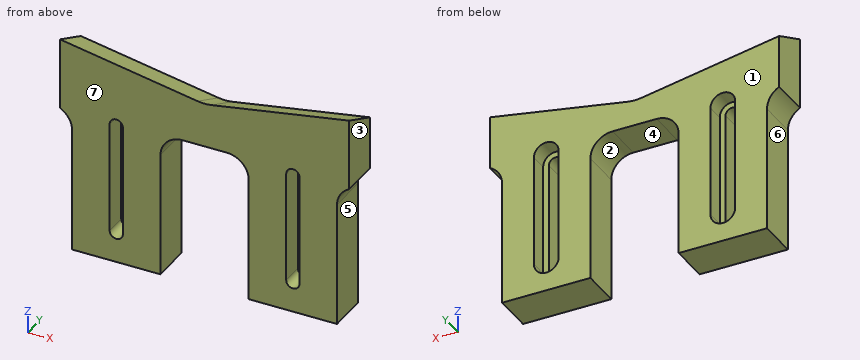
from build123d import *

# Parameters (mm, degrees)
BOSS_EXTRUDE1_DEPTH = 9
CUT_EXTRUDE2_REACH  = 93.001
SKETCH5_W           = 20
SKETCH5_H           = 33.343656478
SKETCH5_W_2         = 7.75
CUT_EXTRUDE3_DEPTH  = 10
FILLET1_R           = 5
CUT_EXTRUDE4_DEPTH  = 4
CHAMFER1_SIZE       = 9
CHAMFER1_SIZE_2     = 4.196768923
FILLET2_R           = 10
CUT_EXTRUDE5_REACH  = 93.001
SKETCH7_W           = 5
SKETCH7_H           = 18.120809616


with BuildPart() as part:
    # Sketch1 → Boss-Extrude1 (new body)
    with BuildSketch(Plane(origin=(0, 0, 0), x_dir=(1, 0, 0), z_dir=(0, 1, 0))):
        Polygon((0, 0), (0, 50), (75.5, 50), (75.5, 0), (37.75, 6.656343522), align=None)
    extrude(amount=BOSS_EXTRUDE1_DEPTH)

    # Sketch4 → Cut-Extrude2 (cut, up to next)
    with BuildSketch(Plane(origin=(0, 9, 0), x_dir=(1, 0, 0), z_dir=(0, 1, 0)), mode=Mode.PRIVATE) as cut_extrude2_sk1:
        with BuildLine():
            Line((19.25, 43), (19.25, 17.656343522))
            ThreePointArc((19.25, 17.656343522), (17.75, 16.156343522), (16.25, 17.656343522))
            Line((16.25, 17.656343522), (16.25, 43))
            ThreePointArc((16.25, 43), (17.75, 44.5), (19.25, 43))
        make_face()
    cut_extrude2_tool1 = extrude(cut_extrude2_sk1.sketch, amount=-CUT_EXTRUDE2_REACH, mode=Mode.PRIVATE) & part.part
    # Sketch4 → Cut-Extrude2 (cut, up to next)
    with BuildSketch(Plane(origin=(0, 9, 0), x_dir=(1, 0, 0), z_dir=(0, 1, 0)), mode=Mode.PRIVATE) as cut_extrude2_sk2:
        with BuildLine():
            Line((59.25, 43), (59.25, 17.656343522))
            ThreePointArc((59.25, 17.656343522), (57.75, 16.156343522), (56.25, 17.656343522))
            Line((56.25, 17.656343522), (56.25, 43))
            ThreePointArc((56.25, 43), (57.75, 44.5), (59.25, 43))
        make_face()
    cut_extrude2_tool2 = extrude(cut_extrude2_sk2.sketch, amount=-CUT_EXTRUDE2_REACH, mode=Mode.PRIVATE) & part.part
    add(cut_extrude2_tool1.solids().sort_by_distance((17.75, 9, -30.328172))[0], mode=Mode.SUBTRACT)
    add(cut_extrude2_tool2.solids().sort_by_distance((57.75, 9, -30.328172))[0], mode=Mode.SUBTRACT)

    # Sketch5 → Cut-Extrude3 (cut)
    with BuildSketch(Plane(origin=(0, 9, 0), x_dir=(1, 0, 0), z_dir=(0, 1, 0))):
        with Locations((37.75, 33.328171761)):
            Rectangle(SKETCH5_W, SKETCH5_H)
        with Locations((71.625, 33.328171761)):
            Rectangle(SKETCH5_W_2, SKETCH5_H)
        with Locations((3.875, 33.328171761)):
            Rectangle(SKETCH5_W_2, SKETCH5_H)
    extrude(amount=-CUT_EXTRUDE3_DEPTH, mode=Mode.SUBTRACT)

    # Fillet1
    fillet1_edges = [part.edges().sort_by_distance(p)[0] for p in [
        (27.75, 4.5, -16.656343522),
        (47.75, 4.5, -16.656343522),
        (7.75, 4.5, -16.656343522),
        (67.75, 4.5, -16.656343522),
    ]]
    fillet(fillet1_edges, radius=FILLET1_R)

    # Sketch6 → Cut-Extrude4 (cut)
    with BuildSketch(Plane(origin=(0, 9, 0), x_dir=(1, 0, 0), z_dir=(0, 1, 0))):
        with BuildLine():
            Line((20.55, 43), (20.55, 17.656343522))
            ThreePointArc((20.55, 17.656343522), (17.75, 14.856343522), (14.95, 17.656343522))
            Line((14.95, 17.656343522), (14.95, 43))
            ThreePointArc((14.95, 43), (17.75, 45.8), (20.55, 43))
        make_face()
        with BuildLine():
            Line((60.55, 43), (60.55, 17.656343522))
            ThreePointArc((60.55, 17.656343522), (57.75, 14.856343522), (54.95, 17.656343522))
            Line((54.95, 17.656343522), (54.95, 43))
            ThreePointArc((54.95, 43), (57.75, 45.8), (60.55, 43))
        make_face()
    extrude(amount=-CUT_EXTRUDE4_DEPTH, mode=Mode.SUBTRACT)

    # Chamfer1
    # the kernel refuses this chamfer: 9, 4.196768923 mm, written as the material it takes off along each edge
    with BuildSketch(Plane(origin=(98.464514589, 9, 4.049263521), x_dir=(-0.0028324039269935573, -0.9998669641130703, 0.01606336089697195), z_dir=(-0.9848077530122074, 0, -0.17364817766693472))) as chamfer1_piece_1_section:
        Polygon((CHAMFER1_SIZE * 0.999866964113, -CHAMFER1_SIZE * 0.0163111641311), (-CHAMFER1_SIZE_2 * 0.0163111641326, -CHAMFER1_SIZE_2 * 0.999866964207), (0, 0), align=None)
    chamfer1_piece_1 = extrude(amount=84.969913084, mode=Mode.PRIVATE)
    chamfer1_piece_1 = split(chamfer1_piece_1, bisect_by=Plane(origin=(68.314499837, 5.890721228, -12.045689495), z_dir=(0.17364817766693472, 0, 0.9848077530122074)), keep=Keep.TOP, mode=Mode.PRIVATE)
    add(chamfer1_piece_1, mode=Mode.SUBTRACT)
    with BuildSketch(Plane(origin=(60.714514589, 9, -10.705607043), x_dir=(0.0028324039269935768, -0.9998669641130703, 0.016063360896972065), z_dir=(-0.9848077530122074, 0, 0.17364817766693472))) as chamfer1_piece_2_section:
        Polygon((CHAMFER1_SIZE * 0.999866964113, -CHAMFER1_SIZE * 0.0163111641311), (-CHAMFER1_SIZE_2 * 0.0163111641326, -CHAMFER1_SIZE_2 * 0.999866964207), (0, 0), align=None)
    chamfer1_piece_2 = extrude(amount=84.969913084, mode=Mode.PRIVATE)
    chamfer1_piece_2 = split(chamfer1_piece_2, bisect_by=Plane(origin=(7.185500163, 5.890721228, -12.045689495), z_dir=(-0.17364817766693472, 0, 0.9848077530122074)), keep=Keep.TOP, mode=Mode.PRIVATE)
    add(chamfer1_piece_2, mode=Mode.SUBTRACT)
    with BuildSketch(Plane(origin=(98.464514589, 9, 4.049263521), x_dir=(-0.0028324039269935573, -0.9998669641130703, 0.01606336089697195), z_dir=(-0.9848077530122074, 0, -0.17364817766693472))) as chamfer1_piece_3a_section:
        Polygon((CHAMFER1_SIZE * 0.999866964113, -CHAMFER1_SIZE * 0.0163111641311), (-CHAMFER1_SIZE_2 * 0.0163111641326, -CHAMFER1_SIZE_2 * 0.999866964207), (0, 0), align=None)
    chamfer1_piece_3a = extrude(amount=84.969913084, mode=Mode.PRIVATE)
    chamfer1_piece_3a = split(chamfer1_piece_3a, bisect_by=Plane(origin=(29.282530451, 6.096120999, -5.163300182), z_dir=(-0.17364817766693472, 0, -0.9848077530122074)), keep=Keep.TOP, mode=Mode.PRIVATE)
    with BuildSketch(Plane(origin=(60.714514589, 9, -10.705607043), x_dir=(0.0028324039269935768, -0.9998669641130703, 0.016063360896972065), z_dir=(-0.9848077530122074, 0, 0.17364817766693472))) as chamfer1_piece_3b_section:
        Polygon((CHAMFER1_SIZE * 0.999866964113, -CHAMFER1_SIZE * 0.0163111641311), (-CHAMFER1_SIZE_2 * 0.0163111641326, -CHAMFER1_SIZE_2 * 0.999866964207), (0, 0), align=None)
    chamfer1_piece_3b = extrude(amount=84.969913084, mode=Mode.PRIVATE)
    chamfer1_piece_3b = split(chamfer1_piece_3b, bisect_by=Plane(origin=(46.217469549, 6.096120999, -5.163300182), z_dir=(0.17364817766693472, 0, -0.9848077530122074)), keep=Keep.TOP, mode=Mode.PRIVATE)
    chamfer1_piece_3 = chamfer1_piece_3a & chamfer1_piece_3b
    add(chamfer1_piece_3, mode=Mode.SUBTRACT)

    # Fillet2
    fillet2_edges = [part.edges().sort_by_distance(p)[0] for p in [
        (37.75, 4.5, -8.787098946),
    ]]
    fillet(fillet2_edges, radius=FILLET2_R)

    # Sketch7 → Cut-Extrude5 (cut, up to next)
    with BuildSketch(Plane(origin=(0, 9, 0), x_dir=(1, 0, 0), z_dir=(0, 1, 0)), mode=Mode.PRIVATE) as cut_extrude5_sk1:
        with Locations((2.5, 9.060404808)):
            Rectangle(SKETCH7_W, SKETCH7_H)
    cut_extrude5_tool1 = extrude(cut_extrude5_sk1.sketch, amount=-CUT_EXTRUDE5_REACH, mode=Mode.PRIVATE) & part.part
    # Sketch7 → Cut-Extrude5 (cut, up to next)
    with BuildSketch(Plane(origin=(0, 9, 0), x_dir=(1, 0, 0), z_dir=(0, 1, 0)), mode=Mode.PRIVATE) as cut_extrude5_sk2:
        with Locations((73, 9.060404808)):
            Rectangle(SKETCH7_W, SKETCH7_H)
    cut_extrude5_tool2 = extrude(cut_extrude5_sk2.sketch, amount=-CUT_EXTRUDE5_REACH, mode=Mode.PRIVATE) & part.part
    add(cut_extrude5_tool1.solids().sort_by_distance((2.5, 9, -9.060405))[0], mode=Mode.SUBTRACT)
    add(cut_extrude5_tool2.solids().sort_by_distance((73, 9, -9.060405))[0], mode=Mode.SUBTRACT)


solid = part.part
Verification items for the finished model (mm, model axes). Face numbers are marked on the shaded views. A direction names the side the tool comes from. Give positions to 0.01 mm unless a question says otherwise; leave off trailing zeros. Write each loop counter-clockwise with the first axis right and the second up, starting at its lowest first coordinate (ties: lowest second). Pieces come first, ordered by that corner, then holes. Notation, with made-up numbers: M 83.5,50.25 L 101.5,50.25 A25 cw 101.5,80.25 Z; hole C 17,11.25 d9. An arc over 180 degrees is marked long. Put each result on its own line as item: value. Start each with the question number.
1. Section check A-A (z = -23). Record the cut outline in (x, y).
2. Section check B-B (x = 57.75). Record the cut outline in (y, z), and give its area (3 significant figures).
3. Set-up check for the marked faces 4, 5, 6 and 7: record each of +Z, -Z, +X, -X, +Y, -Y from which the full face is reachable in a straight line by a thin tool's end or side.
4. Scan lines: line 1 along X through (y, z) = (7, -40.5); line 2 along X through (y, z) = (1.25, -29); line 3 along X through (y, z) = (1, -48). Record each from-to range of solid material in increasing order. Write a range as [from, to].
5. Draft check along X on the marked faces 1, 2 and 3. Enter one of: +X half, -X half, draft (parallel to the pull), parting line (faces both ways), or undercut.
6. Section check D-D (x = 35). Record the cut outline in (y, z).
7. Section check C-C (y = 6.75). Give the number of separate pieces and of enclosed holes in the cut face, and give its area (3 significant figures).
8. Go/stop test with flat-tipped pins: pin 1 Ø4 at (y, z) = (2.5, -34) entering from -X; pin 2 Ø5 at (y, z) = (7.5, -31.5) entering from +X; pin 3 Ø4.5 at (x, y) = (39, 3.5) entering from -Z. Record where each tip stops, or that it passes through.
Answer list:
1. outline: M 7.75,0 L 16.25,0 L 16.25,5 L 14.95,5 L 14.95,9 L 7.75,9 Z; M 19.25,0 L 27.75,0 L 27.75,9 L 20.55,9 L 20.55,5 L 19.25,5 Z; M 47.75,0 L 56.25,0 L 56.25,5 L 54.95,5 L 54.95,9 L 47.75,9 Z; M 59.25,0 L 67.75,0 L 67.75,9 L 60.55,9 L 60.55,5 L 59.25,5 Z
2. outline: M 0,-50 L 9,-50 L 9,-45.8 L 5,-45.8 L 5,-44.5 L 0,-44.5 Z; M 0,-16.16 L 5,-16.16 L 5,-14.86 L 9,-14.86 L 9,-7.39 L 0,-3.13 Z
2. area: 137 mm2
3. face 4: -Z, +Y, -Y
3. face 5: -Z, +X, +Y, -Y
3. face 6: -Z, -X, +Y, -Y
3. face 7: +Z, -Z, +X, -X, -Y
4. line 1: [7.75, 14.95], [20.55, 27.75], [47.75, 54.95], [60.55, 67.75]
4. line 2: [7.75, 16.25], [19.25, 27.75], [47.75, 56.25], [59.25, 67.75]
4. line 3: [7.75, 27.75], [47.75, 67.75]
5. face 1: draft
5. face 2: undercut
5. face 3: +X half
6. outline: M 0,-16.66 L 9,-16.66 L 9,-10.43 L 0,-6.17 Z
7. separate pieces: 1
7. enclosed holes: 2
7. area: 1,660 mm2
8. pin 1: x = 7.75
8. pin 2: x = 67.75
8. pin 3: z = -16.66
